Autodesk Inventor part; units mm, degrees
ref_plane "YZ Plane" through (0, 0, 0) normal (1, 0, 0) x (0, 1, 0)
ref_plane "XZ Plane" through (0, 0, 0) normal (0, 1, 0) x (-1, 0, 0)
ref_plane "XY Plane" through (0, 0, 0) normal (0, 0, 1) x (1, 0, 0)
sketch "스케치3" plane through (0, 0, 0) normal (0, 1, 0) x (-1, 0, 0)
  line L0 (34.9919, -14.4941) -> (14.4941, -34.9919)
  line L1 (14.4941, -34.9919) -> (-14.4941, -34.9919)
  line L2 (-14.4941, -34.9919) -> (-34.9919, -14.4941)
  line L3 (-34.9919, -14.4941) -> (-34.9919, 14.4941)
  line L4 (-34.9919, 14.4941) -> (-14.4941, 34.9919)
  line L5 (-14.4941, 34.9919) -> (14.4941, 34.9919)
  line L6 (14.4941, 34.9919) -> (34.9919, 14.4941)
  line L7 (34.9919, 14.4941) -> (34.9919, -14.4941)
  line L8 (32.5919, -13.5) -> (13.5, -32.5919)
  line L9 (13.5, -32.5919) -> (-13.5, -32.5919)
  line L10 (-13.5, -32.5919) -> (-32.5919, -13.5)
  line L11 (-32.5919, -13.5) -> (-32.5919, 13.5)
  line L12 (-32.5919, 13.5) -> (-13.5, 32.5919)
  line L13 (-13.5, 32.5919) -> (13.5, 32.5919)
  line L14 (13.5, 32.5919) -> (32.5919, 13.5)
  line L15 (32.5919, 13.5) -> (32.5919, -13.5)
  point P0 (0, 0)
  point P1 (0, 0)
  point P2 (0, 0)
  point P3 (0, 0)
  dimension "d43" = 27
  dimension "d44" = 2.4
extrude "돌출2" add sketch "스케치3" along normal blind 3.4 contours L0 L1 L2 L3 L4 L5 L6 L7 | L8 L9 L10 L11 L12 L13 L14 L15
sketch "스케치4" plane through (0, 3.4, 0) normal (0, 1, 0) x (1, 0, 0)
  line L0 (13.5, -32.5919) -> (-13.5, -32.5919)
  line L1 (-13.5, -32.5919) -> (-32.5919, -13.5)
  line L2 (-32.5919, -13.5) -> (-32.5919, 13.5)
  line L3 (-32.5919, 13.5) -> (-13.5, 32.5919)
  line L4 (-13.5, 32.5919) -> (13.5, 32.5919)
  line L5 (13.5, 32.5919) -> (32.5919, 13.5)
  line L6 (32.5919, 13.5) -> (32.5919, -13.5)
  line L7 (32.5919, -13.5) -> (13.5, -32.5919)
  line L8 (-13.9971, 33.7919) -> (13.9971, 33.7919)
  line L9 (13.9971, 33.7919) -> (33.7919, 13.9971)
  line L10 (33.7919, 13.9971) -> (33.7919, -13.9971)
  line L11 (33.7919, -13.9971) -> (13.9971, -33.7919)
  line L12 (13.9971, -33.7919) -> (-13.9971, -33.7919)
  line L13 (-13.9971, -33.7919) -> (-33.7919, -13.9971)
  line L14 (-33.7919, -13.9971) -> (-33.7919, 13.9971)
  line L15 (-33.7919, 13.9971) -> (-13.9971, 33.7919)
  line L16 (-13.1686, 31.7919) -> (13.1686, 31.7919)
  line L17 (13.1686, 31.7919) -> (31.7919, 13.1686)
  line L18 (31.7919, 13.1686) -> (31.7919, -13.1686)
  line L19 (31.7919, -13.1686) -> (13.1686, -31.7919)
  line L20 (13.1686, -31.7919) -> (-13.1686, -31.7919)
  line L21 (-13.1686, -31.7919) -> (-31.7919, -13.1686)
  line L22 (-31.7919, -13.1686) -> (-31.7919, 13.1686)
  line L23 (-31.7919, 13.1686) -> (-13.1686, 31.7919)
  point P0 (0, 0)
  point P1 (0, 0)
  point P2 (0, 0)
  point P3 (0, 0)
  dimension "d7" = 27
  dimension "d42" = 1.2
  dimension "d45" = 0.8
extrude "돌출3" cut sketch "스케치4" against normal blind 1.2 contours L0 L1 L2 L3 L4 L5 L6 L7 | L8 L9 L10 L11 L12 L13 L14 L15 | L16 L17 L18 L19 L20 L21 L22 L23
sketch "스케치5" plane through (0, 0, 0) normal (0, -1, 0) x (1, 0, 0)
  line L0 (10, 2.5) -> (20, 2.5)
  line L1 (20, 2.5) -> (20, -2.5)
  line L2 (20, -2.5) -> (10, -2.5)
  line L3 (10, -2.5) -> (10, 2.5)
  line L4 (10, 2.5) -> (20, -2.5) construction
  line L5 (20, 2.5) -> (10, -2.5) construction
  line L6 (-20, 2.5) -> (-10, 2.5)
  line L7 (-10, 2.5) -> (-10, -2.5)
  line L8 (-10, -2.5) -> (-20, -2.5)
  line L9 (-20, -2.5) -> (-20, 2.5)
  line L10 (-20, 2.5) -> (-10, -2.5) construction
  line L11 (-10, 2.5) -> (-20, -2.5) construction
  point P0 (0, 0)
  point P1 (15, 0)
  point P2 (-15, 0)
  dimension "d11" = 10
  dimension "d12" = 5
  dimension "d13" = 10
  dimension "d16" = 30
extrude "돌출4" add sketch "스케치5" along normal blind 10
sketch "스케치6" plane through (-10, 0, -2.5) normal (0, 0, -1) x (-1, 0, 0)
  circle A0 centre (5, -10) radius 5
  circle A1 centre (-25, -10) radius 5
  line L0 (-20, -10) -> (-30, -10)
  line L1 (10, -10) -> (0, -10)
  point P0 (-10, 0)
  dimension "d23" = 10
  dimension "d24" = 10
extrude "돌출5" add sketch "스케치6" against normal blind 5
sketch "스케치7" plane through (-10, 0, -2.5) normal (0, 0, -1) x (-1, 0, 0)
  circle A0 centre (5, -10) radius 1.25
  line L0 (10, 0) -> (10, -10)
  line L1 (0, 0) -> (10, 0)
  line L2 (4.7788, 0) -> (0, 0)
  circle A1 centre (-25, -10) radius 1.25
  point P0 (-10, 0)
  dimension "d27" = 2.5
  dimension "d28" = 5
  dimension "d31" = 30
extrude "돌출6" cut sketch "스케치7" against normal blind 5
sketch "스케치8" plane through (0, 0, 0) normal (0, -1, 0) x (1, 0, 0)
  circle A0 centre (0, -17.3205) radius 1.25
  line L0 (-10, 2.5) -> (-10, -2.5)
  point P0 (0, 0)
  point P1 (-10, 0)
  dimension "d38" = 2.5
  dimension "d39" = 17.3205
extrude "돌출7" cut sketch "스케치8" against normal blind 5
sketch "스케치9" plane through (0, 2.2, 0) normal (0, 1, 0) x (1, 0, 0)
  line L0 (-13.1686, 31.7919) -> (13.1686, 31.7919)
  line L1 (13.1686, 31.7919) -> (31.7919, 13.1686)
  line L2 (31.7919, 13.1686) -> (31.7919, -13.1686)
  line L3 (31.7919, -13.1686) -> (13.1686, -31.7919)
  line L4 (13.1686, -31.7919) -> (-13.1686, -31.7919)
  line L5 (-13.1686, -31.7919) -> (-31.7919, -13.1686)
  line L6 (-31.7919, -13.1686) -> (-31.7919, 13.1686)
  line L7 (-31.7919, 13.1686) -> (-13.1686, 31.7919)
  line L8 (-13.9971, 33.7919) -> (13.9971, 33.7919)
  line L9 (-11.926, 28.7919) -> (11.926, 28.7919)
  line L10 (11.926, 28.7919) -> (28.7919, 11.926)
  line L11 (28.7919, 11.926) -> (28.7919, -11.926)
  line L12 (28.7919, -11.926) -> (11.926, -28.7919)
  line L13 (11.926, -28.7919) -> (-11.926, -28.7919)
  line L14 (-11.926, -28.7919) -> (-28.7919, -11.926)
  line L15 (-28.7919, -11.926) -> (-28.7919, 11.926)
  line L16 (-28.7919, 11.926) -> (-11.926, 28.7919)
  point P0 (0, 0)
  point P1 (0, 0)
  point P2 (0, 0)
  dimension "d46" = 2
  dimension "d47" = 3
extrude "돌출8" add sketch "스케치9" along normal blind 0.6 contours L0 L1 L2 L3 L4 L5 L6 L7 | L9 L10 L11 L12 L13 L14 L15 L16
fillet "모깎기1" radius 1.2 16 edges at (-34.9919, 3.4, 0) (-24.743, 3.4, 24.743) (0, 3.4, 34.9919) (24.743, 3.4, 24.743) (34.9919, 3.4, 0) (24.743, 3.4, -24.743) (0, 3.4, -34.9919) (-24.743, 3.4, -24.743) (24.743, 0, 24.743) (0, 0, 34.9919) (-24.743, 0, 24.743) (-34.9919, 0, 0) (-24.743, 0, -24.743) (0, 0, -34.9919) (24.743, 0, -24.743) (34.9919, 0, 0)
sketch "스케치10" plane through (0, 0, 0) normal (0, -1, 0) x (1, 0, 0)
  line L0 (-20, 2.5) -> (-10, 2.5)
  line L1 (-10, -2.5) -> (-20, -2.5)
  line L2 (-20, 2.5) -> (-19, 2.5)
  line L3 (-19, 2.5) -> (-19, -2.5)
  line L4 (-19, -2.5) -> (-20, -2.5)
  line L5 (-20, -2.5) -> (-20, 2.5)
  line L6 (20, -2.5) -> (10, -2.5)
  line L7 (10, 2.5) -> (20, 2.5)
  line L8 (20, -2.5) -> (19, -2.5)
  line L9 (19, -2.5) -> (19, 2.5)
  line L10 (19, 2.5) -> (20, 2.5)
  line L11 (20, 2.5) -> (20, -2.5)
  point P0 (0, 0)
  dimension "d54" = 1
  dimension "d55" = 1
extrude "돌출9" cut sketch "스케치10" along normal blind 15
equation "\"d55\" = d54"
properties part number "OV-PAM_top_2"
Geometry: final body of the model. Coordinates: model frame, mm. A direction names the side the tool comes from. Coordinates: 2 decimals unless noted, no trailing zeros. Loops run counter-clockwise (first coordinate to the right, second up) from the corner with the lowest first, then second, coordinate; pieces in that order, holes last. Notation, with made-up numbers: (14.5, 61) - (41.5, 61) arc R22 cw to (41.5, 71) - close; hole circle Ø10 at (70.5, 76). An arc over 180 degrees is marked (long way). One line per question, with ' | ' between items. Start each with the question number.
(1) Cut plane A-A on y = -2. Output: boundary loops of the cut face in (x, z).
(2) Ray query, L1, parallel to Y at x = -15, z = 0.85; L2, parallel to Z at x = 10.5, y = -7; L3, parallel to Y at x = 21, z = 16. Return the intervals inside material, ascending. Write a range as from..to.
(3) Draft query along X for faces 4 (the flat face through (19, -6, 0)), 5 (the cylindrical face through (13.5, -14.77, -0.04)), 6 (the flat face through (14, -7, 2.5)). Return one class per face: +X half, -X half, draft (parallel to the pull), parting line (faces both ways), or undercut.
(4) Reachability of faces 1 (the flat face through (0, 2.2, -17)), 2 (the flat face through (-10, -5, 0)), 3 (the flat face through (-22.61, 2.5, -22.35)) from +Z, -Z, +X, -X, +Y, -Y: full face, straight path, thin tool, end or side. Return the list, or none.
(5) First-contact query: pin 1 (5.5 mm diameter, centred on y = -9.5, z = -0.5, fed in from -X); pin 2 (1 mm diameter, centred on x = -4, z = 22.5, fed in from +Y); pin 3 (1.2 mm diameter, centred on x = 0.5, z = -18, fed in from -Y). Flat tips, straight axial feed; report the tip coordinate or a pass-through.
Here are the results:
1) outline: (-19, -2.5) - (-10, -2.5) - (-10, 2.5) - (-19, 2.5) - close; (10, -2.5) - (19, -2.5) - (19, 2.5) - (10, 2.5) - close
2) L1: -15..-11.25, -8.75..2.8 | L2: -2.5..2.5 | L3: 0..2.8
3) face 4: +X half | face 5: undercut | face 6: draft
4) face 1: -Y | face 2: +Z, -Z, -Y | face 3: +Y
5) pin 1: x = -19 | pin 2: y = 2.8 | pin 3: y = 0
